Work out the finished part from the listing and answer in its coordinate system (mm). A direction names the side the tool comes from. Give positions to 0.01 mm unless a question says otherwise; leave off trailing zeros. Loops run counter-clockwise (first coordinate to the right, second up) from the corner with the lowest first, then second, coordinate; pieces in that order, holes last. Notation, with made-up numbers: M -8,38.25 L 39,38.25 A20 ccw 39,61.25 Z; hole C -15.5,43.25 d1. An arc over 180 degrees is marked long. Use a Markdown table: item, result.
```python
from build123d import *

# Parameters (mm, degrees)
SKETCH_R        = 2.3622
SKETCH_R_2      = 17.78
PAD_DEPTH       = 2.3622
FILLET_R        = 6.35
FILLET001_R     = 6.35
FILLET002_R     = 6.35
FILLET003_R     = 6.35
FILLET004_R     = 6.35
FILLET005_R     = 3.175
FILLET006_R     = 3.175
FILLET007_R     = 6.35
FILLET008_R     = 6.35
FILLET009_R     = 6.35
FILLET010_R     = 6.35
FILLET011_R     = 6.35
FILLET012_R     = 3.175
FILLET013_R     = 3.175
SKETCH001_R     = 1.651
POCKET_DEPTH    = 2.3632
SKETCH002_R     = 2.2479
POCKET001_DEPTH = 2.3632
SKETCH003_R     = 2.2479
POCKET002_DEPTH = 5.0038
SKETCH004_R     = 2.2479
POCKET003_DEPTH = 0.001


with BuildPart() as part:
    # Sketch (on DatumPlane) → Pad (new body)
    with BuildSketch(Plane.XY.offset(43.6758)):
        Polygon((40.4368, 73.025), (-40.4368, 73.025), (-40.4368, 127), (-65.8368, 127), (-197.6882, 22.225), (-197.6882, -22.225), (-65.8368, -127), (-40.4368, -127), (-40.4368, -73.025), (40.4368, -73.025), (40.4368, -127), (72.1868, -127), (72.1868, 127), (40.4368, 127), align=None)
        with Locations((-21.3868, 66.675)):
            Circle(SKETCH_R, mode=Mode.SUBTRACT)
        with Locations((-21.3868, 53.975)):
            Circle(SKETCH_R, mode=Mode.SUBTRACT)
        with Locations((-21.3868, -53.975)):
            Circle(SKETCH_R, mode=Mode.SUBTRACT)
        with Locations((-21.3868, -66.675)):
            Circle(SKETCH_R, mode=Mode.SUBTRACT)
        with Locations((15.0368, 66.675)):
            Circle(SKETCH_R, mode=Mode.SUBTRACT)
        with Locations((15.24, 53.975)):
            Circle(SKETCH_R, mode=Mode.SUBTRACT)
        with Locations((15.24, -53.975)):
            Circle(SKETCH_R, mode=Mode.SUBTRACT)
        with Locations((15.24, -66.675)):
            Circle(SKETCH_R, mode=Mode.SUBTRACT)
        with Locations((-165.9382, 0)):
            Circle(SKETCH_R_2, mode=Mode.SUBTRACT)
    extrude(amount=PAD_DEPTH)

    # Fillet
    fillet_edges = [part.edges().sort_by_distance(p)[0] for p in [
        (-197.6882, -22.225, 44.8569),
    ]]
    fillet(fillet_edges, radius=FILLET_R)

    # Fillet001
    fillet001_edges = [part.edges().sort_by_distance(p)[0] for p in [
        (-65.8368, -127, 44.8569),
    ]]
    fillet(fillet001_edges, radius=FILLET001_R)

    # Fillet002
    fillet002_edges = [part.edges().sort_by_distance(p)[0] for p in [
        (-40.4368, -127, 44.8569),
    ]]
    fillet(fillet002_edges, radius=FILLET002_R)

    # Fillet003
    fillet003_edges = [part.edges().sort_by_distance(p)[0] for p in [
        (-40.4368, -73.025, 44.8569),
    ]]
    fillet(fillet003_edges, radius=FILLET003_R)

    # Fillet004
    fillet004_edges = [part.edges().sort_by_distance(p)[0] for p in [
        (40.4368, -73.025, 44.8569),
    ]]
    fillet(fillet004_edges, radius=FILLET004_R)

    # Fillet005
    fillet005_edges = [part.edges().sort_by_distance(p)[0] for p in [
        (40.4368, -127, 44.8569),
    ]]
    fillet(fillet005_edges, radius=FILLET005_R)

    # Fillet006
    fillet006_edges = [part.edges().sort_by_distance(p)[0] for p in [
        (72.1868, -127, 44.8569),
    ]]
    fillet(fillet006_edges, radius=FILLET006_R)

    # Fillet007
    fillet007_edges = [part.edges().sort_by_distance(p)[0] for p in [
        (-197.6882, 22.225, 44.8569),
    ]]
    fillet(fillet007_edges, radius=FILLET007_R)

    # Fillet008
    fillet008_edges = [part.edges().sort_by_distance(p)[0] for p in [
        (-65.8368, 127, 44.8569),
    ]]
    fillet(fillet008_edges, radius=FILLET008_R)

    # Fillet009
    fillet009_edges = [part.edges().sort_by_distance(p)[0] for p in [
        (-40.4368, 127, 44.8569),
    ]]
    fillet(fillet009_edges, radius=FILLET009_R)

    # Fillet010
    fillet010_edges = [part.edges().sort_by_distance(p)[0] for p in [
        (40.4368, 73.025, 44.8569),
    ]]
    fillet(fillet010_edges, radius=FILLET010_R)

    # Fillet011
    fillet011_edges = [part.edges().sort_by_distance(p)[0] for p in [
        (-40.4368, 73.025, 44.8569),
    ]]
    fillet(fillet011_edges, radius=FILLET011_R)

    # Fillet012
    fillet012_edges = [part.edges().sort_by_distance(p)[0] for p in [
        (40.4368, 127, 44.8569),
    ]]
    fillet(fillet012_edges, radius=FILLET012_R)

    # Fillet013
    fillet013_edges = [part.edges().sort_by_distance(p)[0] for p in [
        (72.1868, 127, 44.8569),
    ]]
    fillet(fillet013_edges, radius=FILLET013_R)

    # Sketch001 (on Face39 of Fillet013) → Pocket (cut, through all)
    with BuildSketch(Plane.XY.offset(46.038)):
        with Locations((-26.2382, 0)):
            Circle(SKETCH001_R)
        with Locations((-34.2011, 0)):
            Circle(SKETCH001_R)
        with Locations((-26.2382, 9.525)):
            Circle(SKETCH001_R)
        with Locations((-18.2753, 0)):
            Circle(SKETCH001_R)
        with Locations((-26.2382, -9.525)):
            Circle(SKETCH001_R)
    extrude(amount=-POCKET_DEPTH, mode=Mode.SUBTRACT)

    # Sketch002 (on Face44 of Pocket) → Pocket001 (cut, through all)
    with BuildSketch(Plane.XY.offset(46.038)):
        with Locations((-96.923253, -96.214243)):
            Circle(SKETCH002_R)
        with Locations((-72.065864, -115.967033)):
            Circle(SKETCH002_R)
        with Locations((-72.065864, 115.967033)):
            Circle(SKETCH002_R)
        with Locations((-96.923253, 96.214243)):
            Circle(SKETCH002_R)
    extrude(amount=-POCKET001_DEPTH, mode=Mode.SUBTRACT)

    # Sketch003 (on Face48 of Pocket001) → Pocket002 (cut)
    with BuildSketch(Plane.XY.offset(46.038)):
        with Locations((67.4243, -117.475)):
            Circle(SKETCH003_R)
        with Locations((67.4243, -66.675)):
            Circle(SKETCH003_R)
        with Locations((67.4243, 117.475)):
            Circle(SKETCH003_R)
        with Locations((67.4243, 66.675)):
            Circle(SKETCH003_R)
    extrude(amount=-POCKET002_DEPTH, mode=Mode.SUBTRACT)

    # Sketch004 → Pocket003 (cut, through all)
    with BuildSketch(Plane.XY):
        with Locations((-177.3809, 19.819338)):
            Circle(SKETCH004_R)
        with Locations((-177.3809, -19.819338)):
            Circle(SKETCH004_R)
        with Locations((-143.0528, 0)):
            Circle(SKETCH004_R)
    extrude(amount=-POCKET003_DEPTH, mode=Mode.SUBTRACT)


solid = part.part
```
(1) Consider probe 1 along X at (y, z) = (52, 45.05); probe 2 along X at (y, z) = (53.5, 44.35); probe 3 along X at (y, z) = (76, 45.55). Determine where each line is inside the solid, lowest interval first. Write a range as [from, to].
Entries:
| item | result |
|---|---|
| probe 1 | x = [-160.22, -22.68], [-20.09, 13.94], [16.54, 72.19] |
| probe 2 | x = [-158.33, -23.7], [-19.07, 12.93], [17.55, 72.19] |
| probe 3 | x = [-130.02, -39.47], [39.47, 72.19] |
(2) A cutting plane is placed at D-D (y = 31). Write down the section's boundary in (x, z).
Entries:
| item | result |
|---|---|
| outline | M -186.65,43.68 L 72.19,43.68 L 72.19,46.04 L -186.65,46.04 Z |
(3) Which of the six approach directions +Z, -Z, +X, -X, +Y, -Y give full straight-line access (tool end or side, diameter ignored) to faces 1 (the flat face through (-35, 2, 46.038)), 2 (the cylindrical face through (38.53, 74.84, 44.87)), 3 (the cylindrical face through (38.53, -74.84, 44.87))?
Entries:
| item | result |
|---|---|
| face 1 | +Z, +X, -X, +Y, -Y |
| face 2 | +Z, -Z, +Y |
| face 3 | +Z, -Z, -Y |
(4) A cutting plane is placed at C-C (x = 9). Write down the section's boundary in (y, z) (3 decimals).
Entries:
| item | result |
|---|---|
| outline | M -73.025,43.676 L 73.025,43.676 L 73.025,46.038 L -73.025,46.038 Z |
(5) A cutting plane is placed at B-B (y = -83.5). Write down the section's boundary in (x, z).
Entries:
| item | result |
|---|---|
| outline | M -120.58,43.68 L -40.44,43.68 L -40.44,46.04 L -120.58,46.04 Z; M 40.44,43.68 L 72.19,43.68 L 72.19,46.04 L 40.44,46.04 Z |
(6) Given P1, Ø1, axis at y = -64.5, z = 44, coming from the -X side; P2, Ø0.7, axis at y = 100.5, z = 45, coming from the -X side, each flat-ended and moving along its own axis, determine where each tip first touches the part or whether it passes through.
Entries:
| item | result |
|---|---|
| P1 | stops at x = -145.12 |
| P2 | stops at x = -99.63 |
(7) A cutting plane is placed at A-A (x = -161.5). Write down the section's boundary in (y, z), and give its area (3 significant figures).
Entries:
| item | result |
|---|---|
| outline | M -50.98,43.68 L -17.22,43.68 L -17.22,46.04 L -50.98,46.04 Z; M 17.22,43.68 L 50.98,43.68 L 50.98,46.04 L 17.22,46.04 Z |
| area | 160 mm² |
